from build123d import *

# Parameters (mm, degrees)
F0_W     = 152.4
F0_H     = 66.675
F1_DEPTH = 6.35
F2_W     = 101.6
F2_H     = 66.675
F3_DEPTH = 101.6
F4_R     = 6.35
F5_W     = 82.55
F5_H     = 47.625
F6_DEPTH = 88.9


with BuildPart() as f1:
    # F0 (on Front) → F1 (new body)
    with BuildSketch(Plane.XZ):
        Rectangle(F0_W, F0_H)
    extrude(amount=F1_DEPTH)

    # F2 (on face) → F3 (join)
    with BuildSketch(Plane.XZ.offset(6.35)):
        Rectangle(F2_W, F2_H)
    extrude(amount=F3_DEPTH)

    # F4
    f4_edges = [f1.edges().sort_by_distance(p)[0] for p in [
        (76.2, -3.175, -33.3375),
        (76.2, -3.175, 33.3375),
        (-76.2, -3.175, 33.3375),
        (-76.2, -3.175, -33.3375),
        (50.8, -57.15, -33.3375),
        (50.8, -57.15, 33.3375),
        (-50.8, -57.15, 33.3375),
        (-50.8, -57.15, -33.3375),
    ]]
    fillet(f4_edges, radius=F4_R)

    # F5 (on face) → F6 (cut)
    with BuildSketch(Plane.XZ.offset(107.95)):
        Rectangle(F5_W, F5_H)
    extrude(amount=-F6_DEPTH, mode=Mode.SUBTRACT)


solid = f1.part
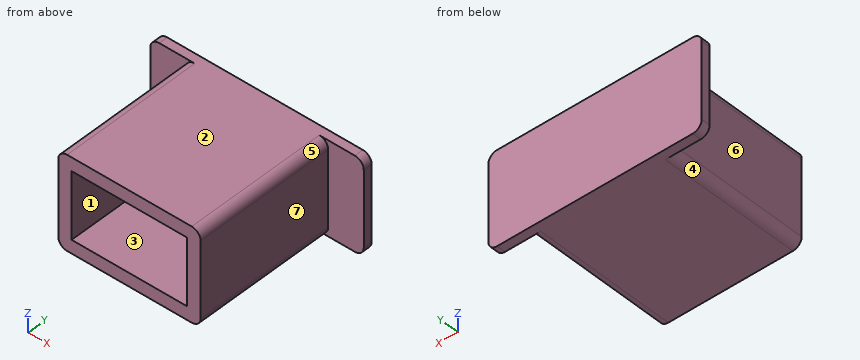
Source: CAD feature listing. Evaluate the final solid. Frame: model axes, mm. Face numbers are marked on the shaded views. A direction names the side the tool comes from. Round coordinates to 2 decimals unless told otherwise and drop trailing zeros. Loops run counter-clockwise (first coordinate to the right, second up) from the corner with the lowest first, then second, coordinate; pieces in that order, holes last. Notation, with made-up numbers: M 80,-16 L 120,-16 A26 cw 120,9 Z; hole C 55,-24.5 d10. An arc over 180 degrees is marked long. Return JSON: item names as keys, results as strings. Group by question number.
1. Mould query, pull axis X, two halves, no side actions, for the marked faces 1, 2, 3 and 4. Classes: released by +X, released by -X, zero draft, split by the parting line, or undercut.
2. Section query C-C on x = 24. Output: boundary loops of the cut face in (y, z).
3. Section query D-D on y = -13.5. Output: boundary loops of the cut face in (x, z).
4. Material intervals for line 1 along X through (y, z) = (-99, 16) (3 decimals); line 2 along Z through (x, y) = (35.5, -71.5); line 3 along Y through (x, z) = (69, -13.5), sorted ascending. Write a range as from..to.
5. Section query B-B on z = 5.5. Output: boundary loops of the cut face in (x, y) (3 decimals), and give its area (3 significant figures).
6. Pin query (flat end, axial travel): pin 1 (5 mm diameter, centred on y = -13.5, z = 25, fed in from -X); pin 2 (3 mm diameter, centred on y = -57, z = -26, fed in from +X); pin 3 (24 mm diameter, centred on x = -2, z = -10, fed in from -Y). Return the tip coordinate at first contact, or that it passes through.
7. Reachability of the marked faces 5, 6 and 7 from +Z, -Z, +X, -X, +Y, -Y: full face, straight path, thin tool, end or side. Return the list, or none.
Checks:
{
 "1": {"face 1": "undercut", "face 2": "zero draft", "face 3": "undercut", "face 4": "released by -X"},
 "2": {"outline": "M -107.95,-33.34 L 0,-33.34 L 0,33.34 L -107.95,33.34 L -107.95,23.81 L -19.05,23.81 L -19.05,-23.81 L -107.95,-23.81 Z"},
 "3": {"outline": "M -50.8,-26.99 A6.35 ccw -44.45,-33.34 L 44.45,-33.34 A6.35 ccw 50.8,-26.99 L 50.8,26.99 A6.35 ccw 44.45,33.34 L -44.45,33.34 A6.35 ccw -50.8,26.99 Z"},
 "4": {"line 1": "x = -50.8..-41.275, 41.275..50.8", "line 2": "z = -33.34..-23.81, 23.81..33.34", "line 3": "y = -6.35..0"},
 "5": {"outline": "M -76.2,-6.35 L -50.8,-6.35 L -50.8,-107.95 L -41.275,-107.95 L -41.275,-19.05 L 41.275,-19.05 L 41.275,-107.95 L 50.8,-107.95 L 50.8,-6.35 L 76.2,-6.35 L 76.2,0 L -76.2,0 Z", "area": "3,950 mm²"},
 "6": {"pin 1": "stops at x = -50.8", "pin 2": "stops at x = 50.8", "pin 3": "stops at y = -19.05"},
 "7": {"face 5": "+Z, +X, -Y", "face 6": "+Z, -Z, -X, -Y", "face 7": "+Z, -Z, +X, -Y"}
}
